Can you work these out from the model? Positions are in its coordinate system, mm. Coordinates: 2 decimals unless noted, no trailing zeros. Loops run counter-clockwise (first coordinate to the right, second up) from the corner with the lowest first, then second, coordinate; pieces in that order, holes last.
```python
from build123d import *

# Parameters (mm, degrees)
EXTRUDE_1_DEPTH = 1
FILLET_1_R      = 4
FILLET_2_R      = 1


with BuildPart() as part:
    # Эскиз1 → Бобышка-Вытянуть1 (new body)
    with BuildSketch(Plane.XY):
        Polygon((0, 0), (29, 7.770526581), (29, 23.299669287), (0, 15.529142706), align=None)
    extrude(amount=EXTRUDE_1_DEPTH)

    # Скругление1
    fillet_1_edges = [part.edges().sort_by_distance(p)[0] for p in [
        (0, 15.529142706, 0.5),
        (29, 23.299669287, 0.5),
        (29, 7.770526581, 0.5),
        (0, 0, 0.5),
    ]]
    fillet(fillet_1_edges, radius=FILLET_1_R)

    # Скругление2
    fillet_2_edges = [part.edges().sort_by_distance(p)[0] for p in [
        (27.435045716, 21.260181156, 1),
        (29, 14.463301164, 1),
        (28.173413361, 8.404788816, 1),
        (15.53527618, 4.162664707, 1),
        (1.564954284, 2.03948813, 1),
        (0, 8.836368123, 1),
        (0.826586639, 14.89488047, 1),
        (13.46472382, 19.13700458, 1),
    ]]
    fillet(fillet_2_edges, radius=FILLET_2_R - 0.0001)  # a hair under: the kernel refuses the full size


solid = part.part
```
Item 1: I need wall thicknesses on line 1 along Y through (x, z) = (12.75, 0.85); line 2 along Y through (x, z) = (14.5, 0.1); line 3 along X through (y, z) = (11, 0.8). Which ranges of each line are inside material? Lowest first, please.
Results are:
line 1: y = 3.91 to 18.46
line 2: y = 3.89 to 19.41
line 3: x = 0.4 to 28.6
Item 2: We'd pull the mould along X, two halves only. Please class faces 1 (the face through (15.604, 4.492, 0.715)), 2 (the face through (13.396, 18.807, 0.715)), 3 (the face through (14, 12, 0)): +X half, -X half, draft (parallel to the pull), parting line (faces both ways), or undercut.
Results are:
face 1: +X half
face 2: -X half
face 3: draft
Item 3: Suppose I cut it at A-A, the plane z = 0.55. Please give me the cut outline in (x, y).
Results are:
outline: (0.16, 5.21) arc R3.84 ccw to (4.99, 1.51) - (25.99, 7.14) arc R3.84 ccw to (28.84, 10.84) - (28.84, 18.09) arc R3.84 ccw to (24.01, 21.79) - (3.01, 16.16) arc R3.84 ccw to (0.16, 12.46) - close
Item 4: I'm going to push a flat-ended pin straight in: P1, Ø5, axis at x = 7, y = 13.5, coming from the -Z side. Where does the tip first touch, or does it pass through?
Results are:
P1: stops at z = 0
